Build history of the part. All positions in model axes, mm. Face numbers are marked on the shaded views. A direction names the side the tool comes from. Round coordinates to 2 decimals unless told otherwise and drop trailing zeros. Order: outer loops, then holes, each group sorted by start corner. A loop starts at its lowest first (then second) coordinate and runs counter-clockwise, first axis right, second up. Notation, with made-up numbers: (60, 15.25) - (66, 15.25) arc R20 cw to (66, 50.25) - close; hole circle Ø8 at (49.25, 83). An arc over 180 degrees is marked (long way). One line per question, with ' | ' between items. Start each with the question number.
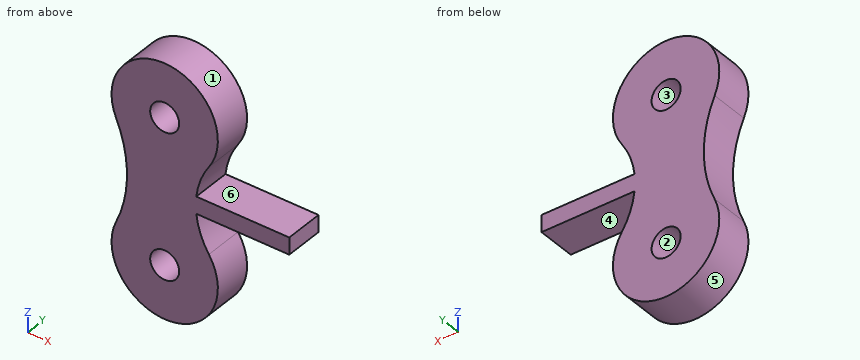
from build123d import *

# Parameters (mm, degrees)
SKETCH1_R           = 1.5
BOSS_EXTRUDE1_DEPTH = 4


with BuildPart() as part:
    # Sketch1 → Boss-Extrude1 (new body)
    with BuildSketch(Plane(origin=(0, 0, 0), x_dir=(1, 0, 0), z_dir=(0, 1, 0))):
        with BuildLine():
            Line((3.268994099, -6.625644187), (12.886719117, -6.625644187))
            Line((12.886719117, -6.625644187), (12.886719117, -8.374355813))
            Line((12.886719117, -8.374355813), (3.268994099, -8.374355813))
            ThreePointArc((3.268994099, -8.374355813), (3.704492519, -10.235637907), (4.570133689, -11.939954566))
            ThreePointArc((4.570133689, -11.939954566), (0.465944189, -20.480227734), (-5.021146674, -12.755431873))
            ThreePointArc((-5.021146674, -12.755431873), (-3.899959484, -7.5), (-5.021146674, -2.244568127))
            ThreePointArc((-5.021146674, -2.244568127), (0.465944189, 5.480227734), (4.570133689, -3.060045434))
            ThreePointArc((4.570133689, -3.060045434), (3.704492519, -4.764362093), (3.268994099, -6.625644187))
        make_face()
        Circle(SKETCH1_R, mode=Mode.SUBTRACT)
        with Locations((0, -15)):
            Circle(SKETCH1_R, mode=Mode.SUBTRACT)
    extrude(amount=BOSS_EXTRUDE1_DEPTH)


solid = part.part
Item 1: Slice it at A-A (z = 0). Write the cut outline in (x, y).
Item 2: Slice it at D-D (x = 7.25). Write the cut outline in (y, z).
Item 3: 3-axis set-ups, long thin cutter, end or side, ignore diameter. For the marked faces 5 and 6: which of +Z, -Z, +X, -X, +Y, -Y reach the whole face in a straight line?
Item 4: Pull direction X, two halves, no side cores. Call the marked faces 1, 2, 3 and 4: released by +X, released by -X, zero draft, split by the parting line, or undercut.
Item 5: Pin check, flat tips, straight feed: pin 1 (2 mm diameter, centred on y = 1, z = 0.5, fed in from -X); pin 2 (1.5 mm diameter, centred on x = -3, y = 1, fed in from +Z); pin 3 (1.8 mm diameter, centred on x = 0, z = 15, fed in from +Y); pin 4 (2 mm diameter, centred on x = 7.5, y = 2.5, fed in from -Z). Stop position of each tip, or through.
Item 6: Wall check: line 1 along Z through (x, y) = (0, 2.5); line 2 along X through (y, z) = (2.75, 0); line 3 along Z through (x, y) = (7.5, 2.75). Give the ranges that are in metal, low to high. Write a range as [from, to].
Item 7: Slice it at B-B (x = 0). Write the cut outline in (y, z).
Item 8: Slice it at C-C (y = 1). Write the cut outline in (x, z).
A:
1) outline: (-5.5, 0) - (-1.5, 0) - (-1.5, 4) - (-5.5, 4) - close; (1.5, 0) - (5.5, 0) - (5.5, 4) - (1.5, 4) - close
2) outline: (0, 6.63) - (4, 6.63) - (4, 8.37) - (0, 8.37) - close
3) face 5: +Y, -Y | face 6: +X, +Y, -Y
4) face 1: split by the parting line | face 2: undercut | face 3: undercut | face 4: zero draft
5) pin 1: x = -5.5 | pin 2: z = 20.02 | pin 3: through | pin 4: z = 6.63
6) line 1: [-5.5, -1.5], [1.5, 13.5], [16.5, 20.5] | line 2: [-5.5, -1.5], [1.5, 5.5] | line 3: [6.63, 8.37]
7) outline: (0, -5.5) - (4, -5.5) - (4, -1.5) - (0, -1.5) - close; (0, 1.5) - (4, 1.5) - (4, 13.5) - (0, 13.5) - close; (0, 16.5) - (4, 16.5) - (4, 20.5) - (0, 20.5) - close
8) outline: (-5.02, 2.24) arc R5.5 ccw (long way) to (4.57, 3.06) arc R7.98 cw to (3.27, 6.63) - (12.89, 6.63) - (12.89, 8.37) - (3.27, 8.37) arc R7.98 cw to (4.57, 11.94) arc R5.5 ccw (long way) to (-5.02, 12.76) arc R12.88 cw to start; hole circle Ø3 at (0, 0); hole circle Ø3 at (0, 15)
